from build123d import *

# Parameters (mm, degrees)
SKETCH_1_W             = 20
SKETCH_1_H             = 20
SKETCH_1_W_2           = 18
SKETCH_1_H_2           = 18
HS_20X20X1_1_DEPTH     = 116
CUT_EXTRUDE_4_DEPTH    = 37
PATTERN_LINEAR_1_COUNT = 4
PATTERN_LINEAR_1_PITCH = 20
SKETCH_5_R             = 1.5
CUT_EXTRUDE_5_DEPTH    = 31


with BuildPart() as part:
    # 草图1 → Hs 20X20X1(1) (new body)
    with BuildSketch(Plane(origin=(0, 0, 0), x_dir=(1, 0, 0), z_dir=(0, 1, 0))):
        Rectangle(SKETCH_1_W, SKETCH_1_H)
        Rectangle(SKETCH_1_W_2, SKETCH_1_H_2, mode=Mode.SUBTRACT)
    extrude(amount=HS_20X20X1_1_DEPTH)

    # 草图4 → 切除-拉伸4 (cut)
    with BuildSketch(Plane(origin=(0, 0, -10), x_dir=(-1, 0, 0), z_dir=(0, 0, -1))):
        with BuildLine():
            Line((-4.5, 33), (4.5, 33))
            ThreePointArc((4.5, 33), (7.5, 30), (4.5, 27))
            Line((4.5, 27), (-4.5, 27))
            ThreePointArc((-4.5, 27), (-7.5, 30), (-4.5, 33))
        make_face()
    cut_extrude_4 = extrude(amount=-CUT_EXTRUDE_4_DEPTH, mode=Mode.SUBTRACT)

    # 阵列(线性)1: 切除-拉伸4 ×4
    with Locations(*[(0, i * PATTERN_LINEAR_1_PITCH, 0) for i in range(1, PATTERN_LINEAR_1_COUNT)]):
        add(cut_extrude_4, mode=Mode.SUBTRACT)

    # 草图5 → 切除-拉伸5 (cut)
    with BuildSketch(Plane(origin=(0, 0, -10), x_dir=(-1, 0, 0), z_dir=(0, 0, -1))):
        with Locations((-4, 3)):
            Circle(SKETCH_5_R)
        with Locations((4, 3)):
            Circle(SKETCH_5_R)
        with Locations((4, 17)):
            Circle(SKETCH_5_R)
        with Locations((-4, 17)):
            Circle(SKETCH_5_R)
        with Locations((-4, 113)):
            Circle(SKETCH_5_R)
        with Locations((4, 113)):
            Circle(SKETCH_5_R)
        with Locations((-4, 99)):
            Circle(SKETCH_5_R)
        with Locations((4, 99)):
            Circle(SKETCH_5_R)
    extrude(amount=-CUT_EXTRUDE_5_DEPTH, mode=Mode.SUBTRACT)


solid = part.part
Work out the finished part from the listing and answer in its coordinate system (mm). A direction names the side the tool comes from. Give positions to 0.01 mm unless a question says otherwise; leave off trailing zeros. Loops run counter-clockwise (first coordinate to the right, second up) from the corner with the lowest first, then second, coordinate; pieces in that order, holes last. Notation, with made-up numbers: (38.25, -13.5) - (44.25, -13.5) arc R5 cw to (44.25, -6.5) - close; hole circle Ø11 at (23.25, -14). An arc over 180 degrees is marked (long way). Answer in a Markdown table with one row per item.
(1) Consider L1, parallel to Z at x = 3.25, y = 40.5; L2, parallel to X at y = 99, z = 9.6. Determine where each line is inside the solid, lowest interval first. Write a range as [from, to].
Results list:
| item | result |
|---|---|
| L1 | z = [-10, -9], [9, 10] |
| L2 | x = [-10, -5.5], [-2.5, 2.5], [5.5, 10] |
(2) Section D-D (x = 0) is taken. State how many separate pieces and enclosed holes the cut face has, and give its area (3 significant figures).
Results list:
| item | result |
|---|---|
| separate pieces | 10 |
| enclosed holes | 0 |
| area | 184 mm² |
(3) A tool of negligible diameter and unlimited length cuts with its end or side. For faces 4 (the face through (-7.5, 90.1, 9.5)), 5 (the face through (-10, 57, 0)), from which of +Z, -Z, +X, -X, +Y, -Y can it reach the whole face along a straight path? Write none if from no direction.
Results list:
| item | result |
|---|---|
| face 4 | +Z, -Z |
| face 5 | +Z, -Z, -X, +Y, -Y |
(4) Section A-A (y = 50) is taken. Give the vertices of the cut face in (x, z), and give its area (3 significant figures).
Results list:
| item | result |
|---|---|
| outline | (-10, -10) - (-7.5, -10) - (-7.5, -9) - (-9, -9) - (-9, 9) - (-7.5, 9) - (-7.5, 10) - (-10, 10) - close; (7.5, -10) - (10, -10) - (10, 10) - (7.5, 10) - (7.5, 9) - (9, 9) - (9, -9) - (7.5, -9) - close |
| area | 46.0 mm² |
(5) Section B-B (y = 99) is taken. Give the vertices of the cut face in (x, z).
Results list:
| item | result |
|---|---|
| outline | (-10, -10) - (-5.5, -10) - (-5.5, -9) - (-9, -9) - (-9, 9) - (-5.5, 9) - (-5.5, 10) - (-10, 10) - close; (-2.5, -10) - (2.5, -10) - (2.5, -9) - (-2.5, -9) - close; (-2.5, 9) - (2.5, 9) - (2.5, 10) - (-2.5, 10) - close; (5.5, -10) - (10, -10) - (10, 10) - (5.5, 10) - (5.5, 9) - (9, 9) - (9, -9) - (5.5, -9) - close |
(6) For a pull along Y with two mould halves and no side action, classify faces 1 (the face through (7.5, 49.9, 9.5)), 2 (the face through (0, 57, -9)), 3 (the face through (-0.8, 116, 9.6)) as pulls with the +Y half, pulls with the -Y half, needs draft (parallel to the pull), parting line crosses it, or undercut.
Results list:
| item | result |
|---|---|
| face 1 | undercut |
| face 2 | needs draft |
| face 3 | pulls with the +Y half |
(7) Section C-C (z = 3) is taken. Give the vertices of the cut face in (x, y).
Results list:
| item | result |
|---|---|
| outline | (-10, 0) - (-9, 0) - (-9, 116) - (-10, 116) - close; (9, 0) - (10, 0) - (10, 116) - (9, 116) - close |
